```python
from build123d import *

# Parameters (mm, degrees)
SKETCH_1_R      = 3.4
EXTRUDE_1_DEPTH = 725


with BuildPart() as part:
    # 草图1 → 凸台-拉伸1 (new body)
    with BuildSketch(Plane(origin=(0, 0, 0), x_dir=(1, 0, 0), z_dir=(0, 1, 0))):
        with BuildLine():
            Line((-12.8, 4.1), (-12.8, 6.495575748))
            Line((-12.8, 6.495575748), (-7.273393207, 6.495575748))
            Line((-7.273393207, 6.495575748), (-5.8, 5.022182541))
            Line((-5.8, 5.022182541), (-5.8, 0))
            Line((-5.8, 0), (-5.8, -5.022182541))
            Line((-5.8, -5.022182541), (-7.273393207, -6.495575748))
            Line((-7.273393207, -6.495575748), (-12.8, -6.495575748))
            Line((-12.8, -6.495575748), (-12.8, -4.1))
            Line((-12.8, -4.1), (-14, -4.1))
            Line((-14, -4.1), (-14, -5.2))
            Line((-14, -5.2), (-15, -5.2))
            Line((-15, -5.2), (-15, -12.5))
            ThreePointArc((-15, -12.5), (-14.267766953, -14.267766953), (-12.5, -15))
            Line((-12.5, -15), (-5.2, -15))
            Line((-5.2, -15), (-5.2, -14))
            Line((-5.2, -14), (-4.1, -14))
            Line((-4.1, -14), (-4.1, -12.8))
            Line((-4.1, -12.8), (-6.495575748, -12.8))
            Line((-6.495575748, -12.8), (-6.495575748, -7.273393207))
            Line((-6.495575748, -7.273393207), (-5.022182541, -5.8))
            Line((-5.022182541, -5.8), (0, -5.8))
            Line((0, -5.8), (5.022182541, -5.8))
            Line((5.022182541, -5.8), (6.495575748, -7.273393207))
            Line((6.495575748, -7.273393207), (6.495575748, -12.8))
            Line((6.495575748, -12.8), (4.1, -12.8))
            Line((4.1, -12.8), (4.1, -14))
            Line((4.1, -14), (5.2, -14))
            Line((5.2, -14), (5.2, -15))
            Line((5.2, -15), (12.5, -15))
            ThreePointArc((12.5, -15), (14.267766953, -14.267766953), (15, -12.5))
            Line((15, -12.5), (15, -5.2))
            Line((15, -5.2), (14, -5.2))
            Line((14, -5.2), (14, -4.1))
            Line((14, -4.1), (12.8, -4.1))
            Line((12.8, -4.1), (12.8, -6.495575748))
            Line((12.8, -6.495575748), (7.273393207, -6.495575748))
            Line((7.273393207, -6.495575748), (5.8, -5.022182541))
            Line((5.8, -5.022182541), (5.8, 0))
            Line((5.8, 0), (5.8, 5.022182541))
            Line((5.8, 5.022182541), (7.273393207, 6.495575748))
            Line((7.273393207, 6.495575748), (12.8, 6.495575748))
            Line((12.8, 6.495575748), (12.8, 4.1))
            Line((12.8, 4.1), (14, 4.1))
            Line((14, 4.1), (14, 5.2))
            Line((14, 5.2), (15, 5.2))
            Line((15, 5.2), (15, 12.5))
            ThreePointArc((15, 12.5), (14.267766953, 14.267766953), (12.5, 15))
            Line((12.5, 15), (5.2, 15))
            Line((5.2, 15), (5.2, 14))
            Line((5.2, 14), (4.1, 14))
            Line((4.1, 14), (4.1, 12.8))
            Line((4.1, 12.8), (6.495575748, 12.8))
            Line((6.495575748, 12.8), (6.495575748, 7.273393207))
            Line((6.495575748, 7.273393207), (5.022182541, 5.8))
            Line((5.022182541, 5.8), (0, 5.8))
            Line((0, 5.8), (-5.022182541, 5.8))
            Line((-5.022182541, 5.8), (-6.495575748, 7.273393207))
            Line((-6.495575748, 7.273393207), (-6.495575748, 12.8))
            Line((-6.495575748, 12.8), (-4.1, 12.8))
            Line((-4.1, 12.8), (-4.1, 14))
            Line((-4.1, 14), (-5.2, 14))
            Line((-5.2, 14), (-5.2, 15))
            Line((-5.2, 15), (-12.5, 15))
            ThreePointArc((-12.5, 15), (-14.267766953, 14.267766953), (-15, 12.5))
            Line((-15, 12.5), (-15, 5.2))
            Line((-15, 5.2), (-14, 5.2))
            Line((-14, 5.2), (-14, 4.1))
            Line((-14, 4.1), (-12.8, 4.1))
        make_face()
        with Locations(Location((0, 0, 0), (0, 0, 270))):
            Circle(SKETCH_1_R, mode=Mode.SUBTRACT)
        with BuildLine():
            Line((-12, 9.5), (-12, 8.25))
            Line((-12, 8.25), (-8.25, 8.25))
            Line((-8.25, 8.25), (-8.25, 12))
            Line((-8.25, 12), (-9.5, 12))
            ThreePointArc((-9.5, 12), (-11.267766953, 11.267766953), (-12, 9.5))
        make_face(mode=Mode.SUBTRACT)
        with BuildLine():
            Line((9.5, 12), (8.25, 12))
            Line((8.25, 12), (8.25, 8.25))
            Line((8.25, 8.25), (12, 8.25))
            Line((12, 8.25), (12, 9.5))
            ThreePointArc((12, 9.5), (11.267766953, 11.267766953), (9.5, 12))
        make_face(mode=Mode.SUBTRACT)
        with BuildLine():
            Line((12, -9.5), (12, -8.25))
            Line((12, -8.25), (8.25, -8.25))
            Line((8.25, -8.25), (8.25, -12))
            Line((8.25, -12), (9.5, -12))
            ThreePointArc((9.5, -12), (11.267766953, -11.267766953), (12, -9.5))
        make_face(mode=Mode.SUBTRACT)
        with BuildLine():
            Line((-9.5, -12), (-8.25, -12))
            Line((-8.25, -12), (-8.25, -8.25))
            Line((-8.25, -8.25), (-12, -8.25))
            Line((-12, -8.25), (-12, -9.5))
            ThreePointArc((-12, -9.5), (-11.267766953, -11.267766953), (-9.5, -12))
        make_face(mode=Mode.SUBTRACT)
    extrude(amount=EXTRUDE_1_DEPTH)


solid = part.part
```
Check sheet for the modelled part. Datum: model origin and axes. Units: mm. Give positions to 0.01 mm unless a question says otherwise; leave off trailing zeros.
Item 1: Scan lines: L1, parallel to X at y = 638.5, z = -8.5; L2, parallel to X at y = 406, z = -10.25; L3, parallel to X at y = 36, z = -4.5. Record each from-to range of solid material in increasing order.
Item 2: Cross-section at A-A (y = 133). Count the separate pieces of the cut face and the enclosed holes in it, and give its area (3 significant figures).
Item 3: Gauge pin test, flat ends, axial feed: pin 1 (5 mm diameter, centred on x = 0.5, y = 313.5, fed in from -Z); pin 2 (1 mm diameter, centred on x = 1.5, y = 338.5, fed in from +Z); pin 3 (1.3 mm diameter, centred on x = 13.5, y = 274.5, fed in from -Z). Record the tip position at first contact, or that the pin passes through.
Report:
1. L1: x = -15 to -12, -8.25 to -6.5, 6.5 to 8.25, 12 to 15
1. L2: x = -15 to -11.88, -8.25 to -6.5, 6.5 to 8.25, 11.88 to 15
1. L3: x = -14 to -12.8, -5.8 to 5.8, 12.8 to 14
2. separate pieces: 1
2. enclosed holes: 5
2. area: 371 mm2
3. pin 1: stops at z = -5.8
3. pin 2: stops at z = 5.8
3. pin 3: stops at z = -14.98
